Read the model definition and answer for the solid it produces. Units are mm, in the model's axes. Face numbers are marked on the shaded views. A direction names the side the tool comes from. Give positions to 0.01 mm unless a question says otherwise; leave off trailing zeros. Order: outer loops, then holes, each group sorted by start corner. A loop starts at its lowest first (then second) coordinate and runs counter-clockwise, first axis right, second up.
Autodesk Fusion 360 part; units mm, degrees
sketch "out" plane through (0, 0, 0) normal (0, 1, 0) x (1, 0, 0)
  line L0 (0, 0) -> (57, 0)
  line L1 (57, 0) -> (57, -30)
  line L2 (57, -30) -> (0, -30)
  line L3 (0, -30) -> (0, 0)
  line L4 (0, 0) -> (57, 0) construction
  line L5 (57, 0) -> (57, 23) construction
  line L6 (57, 23) -> (0, 23) construction
  line L7 (0, 23) -> (0, 0) construction
  ellipse E0 centre (28.5, 0) end of major axis (57, 0) minor radius 23
  line L8 (0, 0) -> (57, 0)
  line L9 (28.5, -23) -> (28.5, 23)
  point P0 (28.5, 0)
  dimension "d25" = 57
  dimension "d26" = 30
  dimension "d27" = 57
  dimension "d28" = 23
  dimension "d29" = 46
extrude "Extrude4" add sketch "out" along normal blind 23.6
ref_plane "WorkPlane2" through (0, 3, 0) normal (0, 1, 0) x (0, 0, 1)
sketch "inner" plane through (0, 3, 0) normal (0, 1, 0) x (1, 0, 0)
  line L0 (0, 0) -> (3, 0) construction
  line L1 (3, 0) -> (54, 0)
  line L2 (54, 0) -> (54, -50)
  line L3 (54, -50) -> (3, -50)
  line L4 (3, -50) -> (3, 0)
  line L5 (3, 0) -> (54, 0) construction
  line L6 (54, 0) -> (54, 20) construction
  line L7 (54, 20) -> (3, 20) construction
  line L8 (3, 20) -> (3, 0) construction
  ellipse E0 centre (28.5, 0) end of major axis (54, 0) minor radius 20
  line L9 (3, 0) -> (54, 0)
  line L10 (28.5, -20) -> (28.5, 20)
  point P0 (28.5, 0)
  dimension "d33" = 3
  dimension "d34" = 51
  dimension "d35" = 50
  dimension "d36" = 51
  dimension "d37" = 20
extrude "Extrude5" cut sketch "inner" along normal blind 17.6
sketch "Sketch7" plane through (0, 0, 0) normal (0, 1, 0) x (1, 0, 0)
  line L0 (0, 0) -> (6, 0) construction
  line L1 (6, 0) -> (51, 0)
  line L2 (51, 0) -> (51, -50)
  line L3 (51, -50) -> (6, -50)
  line L4 (6, -50) -> (6, 0)
  line L5 (6, 0) -> (51, 0) construction
  line L6 (51, 0) -> (51, 14) construction
  line L7 (51, 14) -> (6, 14) construction
  line L8 (6, 14) -> (6, 0) construction
  ellipse E0 centre (28.5, 0) end of major axis (51, 0) minor radius 14
  line L9 (6, 0) -> (51, 0)
  line L10 (28.5, -14) -> (28.5, 14)
  point P0 (28.5, 0)
  dimension "d40" = 6
  dimension "d41" = 45
  dimension "d42" = 50
  dimension "d43" = 45
  dimension "d44" = 14
extrude "Extrude6" cut sketch "Sketch7" along normal blind 3
equation "height = 50 mm"
equation "thickness = 3 mm"
equation "roundDiameter = 40 mm"
equation "inner = 17.6 mm"
equation "width = 51 mm"
equation "d25 = width + ( 2 * thickness )"
equation "d26 = height - ( roundDiameter / 2 )"
equation "d27 = width + ( 2 * thickness )"
equation "d28 = ( roundDiameter / 2 ) + thickness"
equation "d29 = roundDiameter + ( thickness * 2 )"
equation "d30 = inner + ( 2 * thickness )"
equation "d32 = thickness"
equation "d33 = thickness"
equation "d34 = width"
equation "d35 = height"
equation "d36 = width"
equation "d37 = roundDiameter / 2"
equation "d38 = inner"
equation "d40 = thickness * 2"
equation "d41 = width - ( 2 * thickness )"
equation "d42 = height"
equation "d43 = width - ( 2 * thickness )"
equation "d44 = roundDiameter / 2 - ( 2 * thickness )"
equation "d45 = thickness"
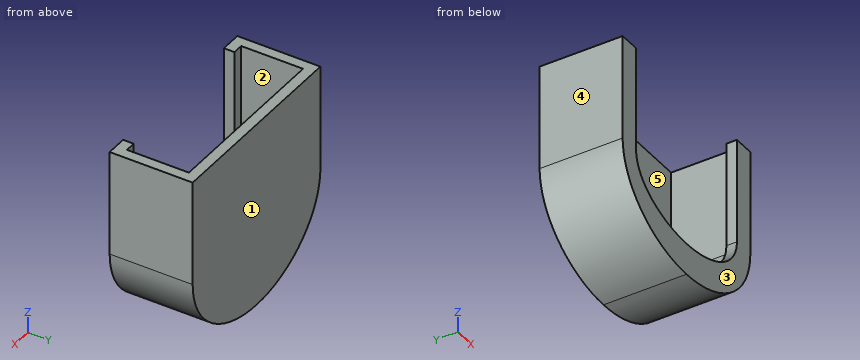
1) Consider L1, parallel to X at y = 11.75, z = 15; L2, parallel to Y at x = 38, z = -9; L3, parallel to X at y = 2.75, z = -8. Determine where each line is inside the solid, lowest interval first.
Final values:
L1: x = 0 to 3, 54 to 57
L2: y = 20.6 to 23.6
L3: x = 1.78 to 10.04, 46.96 to 55.22
2) For a pull along X with two mould halves and no side action, classify the marked faces 3, 4 and 5 as released by +X, released by -X, zero draft, split by the parting line, or undercut.
Final values:
face 3: zero draft
face 4: released by -X
face 5: undercut
3) A tool of negligible diameter and unlimited length cuts with its end or side. For the marked faces 1 and 2, from which of +Z, -Z, +X, -X, +Y, -Y can it reach the whole face along a straight path? Write none if from no direction.
Final values:
face 1: +Z, -Z, +X, -X, +Y
face 2: +Z
4) Given pin 1 (10 mm diameter, centred on x = 38.5, y = 14, fed in from -Z); pin 2 (5 mm diameter, centred on x = 33.5, y = 10.5, fed in from -Z); pin 3 (25 mm diameter, centred on x = 37, z = 6.5, fed in from -Y), each flat-ended and moving along its own axis, determine where each tip first touches the part or whether it passes through.
Final values:
pin 1: stops at z = -22.64
pin 2: stops at z = -22.91
pin 3: stops at y = 20.6
5) The part is cut by section A-A on z = 12. Determine the outline of the cut face in (x, y).
Final values:
outline: (0, 0) - (6, 0) - (6, 3) - (3, 3) - (3, 20.6) - (54, 20.6) - (54, 3) - (51, 3) - (51, 0) - (57, 0) - (57, 23.6) - (0, 23.6) - close
